```python
from build123d import *

# Parameters (mm, degrees)
SKETCH1_R           = 5.87375
SKETCH1_W           = 3.175
SKETCH1_H           = 3.175
BOSS_EXTRUDE1_DEPTH = 3.175


with BuildPart() as part:
    # Sketch1 → Boss-Extrude1 (new body)
    with BuildSketch(Plane(origin=(0, 0, 0), x_dir=(0, 0, -1), z_dir=(1, 0, 0))):
        Circle(SKETCH1_R)
        Rectangle(SKETCH1_W, SKETCH1_H, mode=Mode.SUBTRACT)
    extrude(amount=BOSS_EXTRUDE1_DEPTH)

    # Sketch2 → Cut-Revolve1 (revolve, cut)
    with BuildSketch(Plane.XY, mode=Mode.PRIVATE) as cut_revolve1_sk:
        Polygon((0, 5.87375), (3.175, 5.87375), (3.175, 3.650591066), align=None)
    revolve(cut_revolve1_sk.sketch.rotate(Axis((0, 0, 0), (1, 0, 0)), 90), axis=Axis((0, 0, 0), (1, 0, 0)), mode=Mode.SUBTRACT)


solid = part.part
```
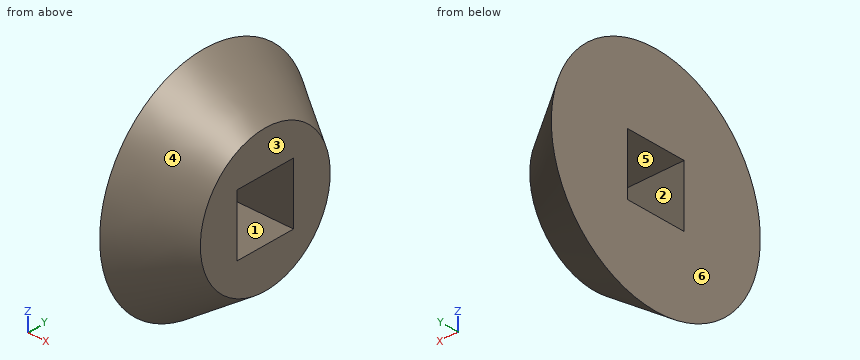
Verification items for the finished model (mm, model axes). Face numbers are marked on the shaded views. A direction names the side the tool comes from. Give positions to 0.01 mm unless a question says otherwise; leave off trailing zeros. Order: outer loops, then holes, each group sorted by start corner. A loop starts at its lowest first (then second) coordinate and runs counter-clockwise, first axis right, second up. Notation, with made-up numbers: (-28.5, -33) -> (13.5, -33) arc R22 cw to (13.5, -5) -> close; hole circle Ø1 at (-32, 32.25). An arc over 180 degrees is marked (long way). One line per item, written item: value.
(1) Gauge pin test, flat ends, axial feed: pin 1 (1 mm diameter, centred on x = 1.5, z = 0.5, fed in from +Y); pin 2 (1.5 mm diameter, centred on x = 0.5, z = -3.5, fed in from +Y); pin 3 (1.6 mm diameter, centred on x = 1, z = -0.5, fed in from -Y). Record the tip position at first contact, or that the pin passes through.
Final values:
pin 1: y = 5.15
pin 2: y = 5.08
pin 3: y = -5.72
(2) Sectioned sample at D-D on x = 0.45. Record the cut outline in (y, z), then the cut area to 3 significant figures.
Final values:
outline: circle Ø11.12 at (0, 0); hole (-1.59, -1.59) -> (1.59, -1.59) -> (1.59, 1.59) -> (-1.59, 1.59) -> close
area: 87.0 mm^2
(3) Scan lines: line 1 along Y through (x, z) = (2.75, 1); line 2 along Z through (x, y) = (0.25, -0.5); line 3 along Z through (x, y) = (1.55, -0.5). Record each from-to range of solid material in increasing order. Write a range as [from, to].
Final values:
line 1: [-3.82, -1.59], [1.59, 3.82]
line 2: [-5.68, -1.59], [1.59, 5.68]
line 3: [-4.76, -1.59], [1.59, 4.76]
(4) Draft check along Z on the marked faces 1, 2, 3 and 4. Enter one of: pulls with the +Z half, pulls with the -Z half, needs draft (parallel to the pull), parting line crosses it, or undercut.
Final values:
face 1: undercut
face 2: undercut
face 3: needs draft
face 4: parting line crosses it
(5) Tool access check on the marked faces 5 and 6. Record the directions out of +Z, -Z, +X, -X, +Y, -Y that give a thin tool (end or side, any length) a straight path to the whole face; none if there is none.
Final values:
face 5: +X, -X
face 6: +Z, -Z, -X, +Y, -Y
(6) Sectioned sample at A-A on y = 0. Record the cut outline in (x, z) (1 decimal), then the cut area to 3 significant figures.
Final values:
outline: (0, -5.9) -> (3.2, -3.7) -> (3.2, -1.6) -> (0, -1.6) -> close; (0, 1.6) -> (3.2, 1.6) -> (3.2, 3.7) -> (0, 5.9) -> close
area: 20.2 mm^2
(7) Sectioned sample at C-C on x = 1.1. Record the cut outline in (y, z).
Final values:
outline: circle Ø10.21 at (0, 0); hole (-1.59, -1.59) -> (1.59, -1.59) -> (1.59, 1.59) -> (-1.59, 1.59) -> close
